Could you check a few things on this model? Use its own coordinates, in mm. Face numbers are marked on the shaded views. Round coordinates to 2 decimals unless told otherwise and drop trailing zeros. Loops run counter-clockwise (first coordinate to the right, second up) from the corner with the lowest first, then second, coordinate; pieces in that order, holes last.
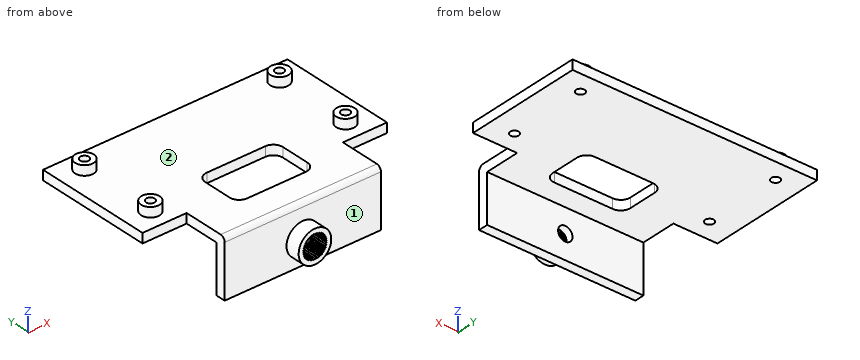
from build123d import *

# Parameters (mm, degrees)
SKETCH1_W               = 51
SKETCH1_H               = 12
BRACKET_SIZE_DEPTH      = 34
SKETCH2_W               = 10
SKETCH2_H               = 32
SIDE_PROFILE_DEPTH      = 45.161634934
SIDE_PROFILE_DEPTH_BACK = 45.161634934
FILLET1_R               = 1
SKETCH3_W               = 9.2
SKETCH3_H               = 9.4
BASE_TRIM_DEPTH         = 45.161634934
WIRE_REILEF_HOLE_DEPTH  = 45.161634934
SKETCH5_R               = 1.95
SPACER_DEPTH            = 2
M1_6_CLEARANCE_HOLE1_D  = 1.8
SKETCH8_R               = 3.4
SERVO_SPACER_DEPTH      = 3
SPLINE_TOOTH_DEPTH      = 3.5
SPLINE_COUNT            = 36
M2_CLEARANCE_HOLE1_D    = 3


with BuildPart() as part:
    # Sketch1 → Bracket Size (new body)
    with BuildSketch(Plane(origin=(0, 0, 0), x_dir=(1, 0, 0), z_dir=(0, 1, 0))):
        with Locations((0, 6)):
            Rectangle(SKETCH1_W, SKETCH1_H)
    extrude(amount=BRACKET_SIZE_DEPTH)

    # Sketch2 → Side Profile (cut, two sides)
    with BuildSketch(Plane(origin=(0, 0, 0), x_dir=(0, 0, -1), z_dir=(1, 0, 0))) as side_profile_sk:
        with Locations((7, 18)):
            Rectangle(SKETCH2_W, SKETCH2_H)
    extrude(amount=SIDE_PROFILE_DEPTH, mode=Mode.SUBTRACT)
    extrude(side_profile_sk.sketch, amount=-SIDE_PROFILE_DEPTH_BACK, mode=Mode.SUBTRACT)

    # Fillet1
    fillet1_edges = [part.edges().sort_by_distance(p)[0] for p in [
        (0, 0, 0),
    ]]
    fillet(fillet1_edges, radius=FILLET1_R)

    # Sketch3 → Base Trim (cut, through all)
    with BuildSketch(Plane.XY):
        with Locations((20.9, 4.7)):
            Rectangle(SKETCH3_W, SKETCH3_H)
        with Locations((-20.9, 4.7)):
            Rectangle(SKETCH3_W, SKETCH3_H)
    extrude(amount=-BASE_TRIM_DEPTH, mode=Mode.SUBTRACT)

    # Sketch4 → Wire Reilef Hole (cut, through all)
    with BuildSketch(Plane.XY):
        with BuildLine():
            Line((-6.1, 16.5), (6.1, 16.5))
            ThreePointArc((6.1, 16.5), (7.514213562, 15.914213562), (8.1, 14.5))
            Line((8.1, 14.5), (8.1, 8.5))
            ThreePointArc((8.1, 8.5), (7.514213562, 7.085786438), (6.1, 6.5))
            Line((6.1, 6.5), (-6.1, 6.5))
            ThreePointArc((-6.1, 6.5), (-7.514213562, 7.085786438), (-8.1, 8.5))
            Line((-8.1, 8.5), (-8.1, 14.5))
            ThreePointArc((-8.1, 14.5), (-7.514213562, 15.914213562), (-6.1, 16.5))
        make_face()
    extrude(amount=-WIRE_REILEF_HOLE_DEPTH, mode=Mode.SUBTRACT)

    # Sketch5 → Spacer (add)
    with BuildSketch(Plane.XY):
        with Locations(Location((-20.35, 29.85, 0), (0, 0, 180))):
            Circle(SKETCH5_R)
    spacer = extrude(amount=SPACER_DEPTH)

    # M1.6 Clearance Hole1 (through all)
    with Locations(Plane.XY.offset(2)):
        with Locations((-20.35, 29.85)):
            m1_6_clearance_hole1 = Hole(M1_6_CLEARANCE_HOLE1_D / 2)

    # Spacer Pattern: Spacer, M1.6 Clearance Hole1 at 3 more places
    with Locations((0, -16.3, 0), (40.7, -16.3, 0), (40.7, 0, 0)):
        add(spacer)
        add(m1_6_clearance_hole1, mode=Mode.SUBTRACT)

    # Sketch8 → Servo Spacer (add)
    with BuildSketch(Plane(origin=(0, 0, 0), x_dir=(1, 0, 0), z_dir=(0, 1, 0))):
        with Locations(Location((0, 7, 0), (0, 0, 270))):
            Circle(SKETCH8_R)
    extrude(amount=-SERVO_SPACER_DEPTH)

    # Sketch9 → Spline Tooth (cut)
    with BuildSketch(Plane.XZ.offset(3)):
        Polygon((0.39070839, -4.78418261), (0.217889353, -4.509513302), (0, -4.750000055), (0, -7), align=None)
    spline_tooth = extrude(amount=-SPLINE_TOOTH_DEPTH, mode=Mode.SUBTRACT)

    # Spline: Spline Tooth ×36 about axis
    spline_axis = Axis((0, 0, -7), (0, 1, 0))
    for i in range(1, SPLINE_COUNT):
        add(spline_tooth.rotate(spline_axis, i * 360 / SPLINE_COUNT), mode=Mode.SUBTRACT)

    # M2 Clearance Hole1 (through all)
    with Locations(Plane.XZ):
        with Locations((0, -7)):
            Hole(M2_CLEARANCE_HOLE1_D / 2)


solid = part.part
Item 1: If we section it at C-C, the plane x = 10: Please give me the cut outline in (y, z).
Results list:
outline: (0, -12) - (2, -12) - (2, -2) - (34, -2) - (34, 0) - (1, 0) arc R1 ccw to (0, -1) - close
Item 2: We'd pull the mould along X, two halves only. Please class the marked faces 1 and 2: released by +X, released by -X, zero draft, split by the parting line, or undercut.
Results list:
face 1: zero draft
face 2: undercut
Item 3: Will these pins go through, and if not, where does the flat tip stop? pin 1 (1.5 mm diameter, centred on x = -11, z = -6, fed in from -Y); pin 2 (3 mm diameter, centred on x = -20.35, y = 29.85, fed in from -Z); pin 3 (1.6 mm diameter, centred on x = 19, z = -0.5, fed in from -Y).
Results list:
pin 1: stops at y = 0
pin 2: stops at z = -2
pin 3: stops at y = 9.4
Item 4: If we section it at B-B, the plane x = 20.35: Please give me the cut outline in (y, z).
Results list:
outline: (9.4, -2) - (12.65, -2) - (12.65, 2) - (11.6, 2) - (11.6, 0) - (9.4, 0) - close; (14.45, -2) - (28.95, -2) - (28.95, 2) - (27.9, 2) - (27.9, 0) - (15.5, 0) - (15.5, 2) - (14.45, 2) - close; (30.75, -2) - (34, -2) - (34, 0) - (31.8, 0) - (31.8, 2) - (30.75, 2) - close
Item 5: If we section it at A-A, the plane y = 11: Please give me the cut outline in (x, z), then the cut area to 3 significant figures.
Results list:
outline: (-25.5, -2) - (-8.1, -2) - (-8.1, 0) - (-25.5, 0) - close; (8.1, -2) - (25.5, -2) - (25.5, 0) - (8.1, 0) - close
area: 69.6 mm2
Item 6: If I drill on line 1 along Z through (x, y) = (11.5, 16); line 2 along Y through (x, z) = (-13.5, -11); line 3 along X through (y, z) = (28.5, 0.5), over which ranges is the centre line in solid material (lowest first)?
Results list:
line 1: z = -2 to 0
line 2: y = 0 to 2
line 3: x = -21.76 to -18.94, 18.94 to 21.76
Item 7: If we section it at D-D, the plane y = 3.5: Please give me the cut outline in (x, z), then the cut area to 3 significant figures.
Results list:
outline: (-16.3, -2) - (16.3, -2) - (16.3, 0) - (-16.3, 0) - close
area: 65.2 mm2
